Model file for the job. Use its own axes, mm. Face numbers are marked on the shaded views. Round coordinates to 2 decimals unless told otherwise and drop trailing zeros. Loops run counter-clockwise (first coordinate to the right, second up) from the corner with the lowest first, then second, coordinate; pieces in that order, holes last. Notation, with made-up numbers: (31.5, 47.5) -> (90.5, 47.5) arc R33 ccw to (90.5, 84.5) -> close; hole circle Ø8 at (36, -13.75). An arc over 180 degrees is marked (long way). Use a Markdown table: item, result.
from build123d import *

# Parameters (mm, degrees)
F0_W     = 60
F0_H     = 100
F1_DEPTH = 51
F2_SIZE  = 20
F4_D     = 10
F4_DEPTH = 12
F4_TIP   = 3.0043030951
F5_R     = 5


with BuildPart() as f1:
    # F0 (on Top) → F1 (new body)
    with BuildSketch(Plane.XY):
        with Locations((30, 50)):
            Rectangle(F0_W, F0_H)
    extrude(amount=F1_DEPTH)

    # F2
    f2_edges = [f1.edges().sort_by_distance(p)[0] for p in [
        (60, 50, 51),
    ]]
    chamfer(f2_edges, length=F2_SIZE)

    # F4
    with Locations(Plane(origin=(45.5, 0, 45.5), x_dir=(0.7071067812, 0, -0.7071067812), z_dir=(0.7071067812, 0, 0.7071067812))):
        with Locations((6.3639610307, 24.4938470423), (6.3639610307, 68.0030360818)):
            Hole(F4_D / 2, depth=F4_DEPTH)
            with Locations((0, 0, -(F4_DEPTH + F4_TIP / 2))):  # 118° drill point
                Cone(0, F4_D / 2, F4_TIP, mode=Mode.SUBTRACT)

    # F5
    f5_edges = [f1.edges().sort_by_distance(p)[0] for p in [
        (30, 100, 0),
        (30, 0, 0),
    ]]
    fillet(f5_edges, radius=F5_R)


solid = f1.part
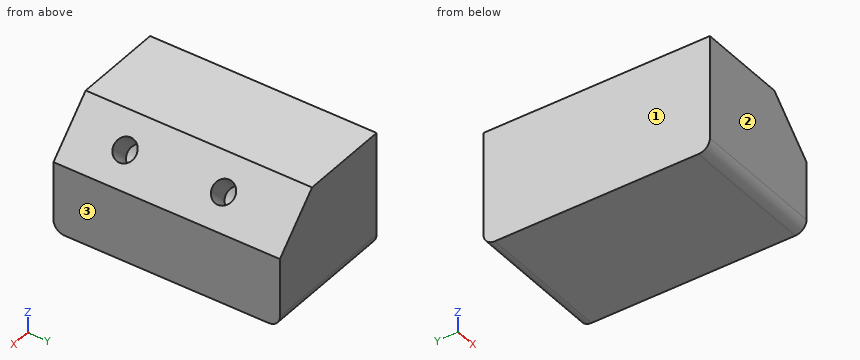
Q1. Flat gauge pins, fed straight in: pin 1 (5 mm diameter, centred on x = 41.5, y = 79, fed in from +Z); pin 2 (4 mm diameter, centred on x = 53, y = 62, fed in from +Z). Where does each tip first touch, or does it go through?
Results list:
| item | result |
|---|---|
| pin 1 | stops at z = 51 |
| pin 2 | stops at z = 40 |
Q2. Band-saw the part on A-A, the plane y = 42. Give the cut face in (x, z).
Results list:
| item | result |
|---|---|
| outline | (0, 0) -> (60, 0) -> (60, 31) -> (40, 51) -> (0, 51) -> close |
Q3. Band-saw the part on B-B, the plane x = 43.5. Give the number of separate pieces and of enclosed holes in the cut face, plus the area to 3 significant figures.
Results list:
| item | result |
|---|---|
| separate pieces | 1 |
| enclosed holes | 2 |
| area | 4,540 mm² |
Q4. Pull direction X, two halves, no side cores. Call the marked faces 1, 2 and 3: released by +X, released by -X, zero draft, split by the parting line, or undercut.
Results list:
| item | result |
|---|---|
| face 1 | released by -X |
| face 2 | zero draft |
| face 3 | released by +X |
Q5. Drill centre lines: L1, parallel to Y at x = 44, z = 36; L2, parallel to Y at x = 39, z = 4.5; L3, parallel to X at y = 34.5, z = 43. Where is each one in solid material? Low to high. Write a range as from..to.
Results list:
| item | result |
|---|---|
| L1 | y = 0..19.54, 29.44..63.05, 72.95..100 |
| L2 | y = 0.03..99.97 |
| L3 | x = 0..48 |
